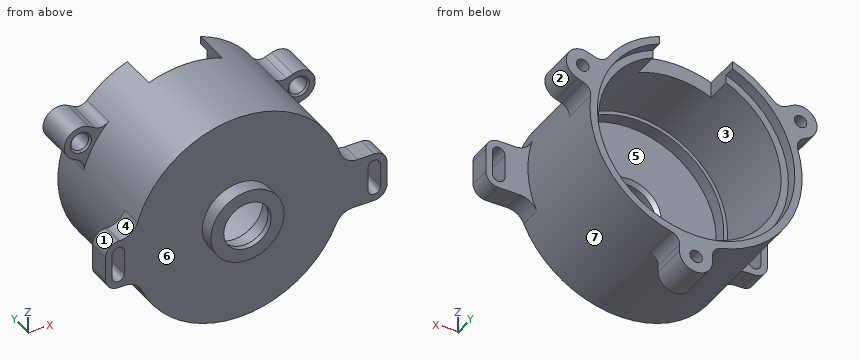
from build123d import *

# Parameters (mm, degrees)
ESQUISSE1_R                        = 2.4
BOSS_EXTRU_1_DEPTH                 = 10
ESQUISSE1_3_R                      = 2.4
BOSS_EXTRU_2_DEPTH                 = 4
CHANFREIN2_SIZE                    = 0.5
CONG_1_R                           = 3
R_P_TITION_START                   = 27.5
R_P_TITION_CIRCULAIRE1_OUTLINE_R   = 2.4
R_P_TITION_CIRCULAIRE1_DEPTH       = 4
R_P_TITION_START_2                 = 21.5
R_P_TITION_CIRCULAIRE1_2_OUTLINE_R = 2.4
R_P_TITION_CIRCULAIRE1_2_DEPTH     = 10
M3_CLEARANCE_HOLE1_D               = 3.4
ENL_V_MAT_EXTRU_2_DEPTH            = 10
BOSS_EXTRU_3_START                 = -6
BOSS_EXTRU_3_DEPTH                 = 6
CONG_3_R                           = 5


with BuildPart() as part:
    # Sketch1 → Revolve1 (revolve)
    with BuildSketch(Plane.XY, mode=Mode.PRIVATE) as revolve1_sk:
        Polygon((29, -3.5), (29, 31.5), (27, 31.5), (27, 28.5), (25, 28.5), (25, 3.5), (24, 3.5), (24, 0), (9, 0), (8, -1), (8, -6), (6.5, -6), (6.5, -7.5), (10, -7.5), (10, -3.5), align=None)
    revolve(revolve1_sk.sketch.rotate(Axis((0, 34.575175177, 0), (0, -1, 0)), 90), axis=Axis((0, 34.575175177, 0), (0, -1, 0)))

    # Esquisse1 → Boss.-Extru.1 (add)
    with BuildSketch(Plane(origin=(0, 31.5, 0), x_dir=(1, 0, 0), z_dir=(0, 1, 0))):
        with BuildLine():
            Line((4.5, 28.648734702), (4.5, 33))
            ThreePointArc((4.5, 33), (0, 37.5), (-4.5, 33))
            Line((-4.5, 33), (-4.5, 28.648734702))
            ThreePointArc((-4.5, 28.648734702), (0, 29), (4.5, 28.648734702))
        make_face()
        with Locations(Location((0, 33, 0), (0, 0, 270))):
            Circle(ESQUISSE1_R, mode=Mode.SUBTRACT)
    extrude(amount=-BOSS_EXTRU_1_DEPTH)

    # Esquisse1<3> → Boss.-Extru.2 (add)
    with BuildSketch(Plane(origin=(0, 31.5, 0), x_dir=(1, 0, 0), z_dir=(0, 1, 0))):
        with Locations(Location((0, 33, 0), (0, 0, 270))):
            Circle(ESQUISSE1_3_R)
    extrude(amount=-BOSS_EXTRU_2_DEPTH)

    # Chanfrein2
    chanfrein2_edges = [part.edges().sort_by_distance(p)[0] for p in [
        (0, 21.5, -35.4),
    ]]
    chamfer(chanfrein2_edges, length=CHANFREIN2_SIZE)

    # Congé1
    cong_1_edges = [part.edges().sort_by_distance(p)[0] for p in [
        (4.5, 26.5, -28.648734702),
        (-4.5, 26.5, -28.648734702),
    ]]
    fillet(cong_1_edges, radius=CONG_1_R)



with BuildPart() as body_2:
    # Répétition circulaire1: read off the stored shape, not the designer's step
    # Répétition circulaire1 outline → Répétition circulaire1 (new body)
    with BuildSketch(Plane(origin=(0, 0, 0), x_dir=(1, 0, 0), z_dir=(0, 1, 0)).offset(R_P_TITION_START)):
        with Locations((31.009856486, -11.28666473)):
            Circle(R_P_TITION_CIRCULAIRE1_OUTLINE_R)
        with Locations((-28.578838325, -16.5)):
            Circle(R_P_TITION_CIRCULAIRE1_OUTLINE_R)
    extrude(amount=R_P_TITION_CIRCULAIRE1_DEPTH)


with BuildPart() as part_1:
    add(part.part)

    add(body_2.part)  # R_p_tition circulaire1 2 merges body 2
    # R_p_tition circulaire1 2 outline → R_p_tition circulaire1 2 (add)
    # profile 1 of 2: a face of its own
    with BuildSketch(Plane(origin=(0, 0, 0), x_dir=(1, 0, 0), z_dir=(0, 1, 0)).offset(R_P_TITION_START_2)):
        with BuildLine():
            Line((-29.190907557, -11.657225913), (-30.828838325, -12.602885683))
            ThreePointArc((-30.828838325, -12.602885683), (-32.475952642, -18.75), (-26.328838325, -20.397114317))
            Line((-26.328838325, -20.397114317), (-24.690907557, -19.451454547))
            ThreePointArc((-24.690907557, -19.451454547), (-22.761849141, -19.080371134), (-21.016759974, -19.98238725))
            ThreePointArc((-21.016759974, -19.98238725), (-25.11473671, -14.5), (-27.813634974, -8.209854417))
            ThreePointArc((-27.813634974, -8.209854417), (-27.905010686, -10.172154026), (-29.190907557, -11.657225913))
        make_face()
        with Locations((-28.578838325, -16.5)):
            Circle(R_P_TITION_CIRCULAIRE1_2_OUTLINE_R, mode=Mode.SUBTRACT)
    # profile 2 of 2: a face of its own
    with BuildSketch(Plane(origin=(0, 0, 0), x_dir=(1, 0, 0), z_dir=(0, 1, 0)).offset(R_P_TITION_START_2)):
        with BuildLine():
            ThreePointArc((30.771688116, -6.411178556), (29.247446881, -5.171961896), (28.81670962, -3.255341254))
            ThreePointArc((28.81670962, -3.255341254), (27.251086003, -9.918584157), (24.167373297, -16.029287818))
            ThreePointArc((24.167373297, -16.029287818), (25.729317183, -14.8379438), (27.693506826, -14.868412143))
            Line((27.693506826, -14.868412143), (29.470765841, -15.515281523))
            ThreePointArc((29.470765841, -15.515281523), (35.238473279, -12.825755374), (32.548947131, -7.058047936))
            Line((32.548947131, -7.058047936), (30.771688116, -6.411178556))
        make_face()
        with Locations((31.009856486, -11.28666473)):
            Circle(R_P_TITION_CIRCULAIRE1_2_OUTLINE_R, mode=Mode.SUBTRACT)
    extrude(amount=R_P_TITION_CIRCULAIRE1_2_DEPTH)

    # R_p_tition circulaire1 3: loft between two sections, ruled curve by curve
    r_p_tition_circulaire1_3_from = [
        Edge.make_three_point_arc((-28.578838325, 22, 18.9), (-30.978838325, 22, 16.5), (-28.578838325, 22, 14.1)),
        Edge.make_three_point_arc((-28.578838325, 22, 14.1), (-26.178838325, 22, 16.5), (-28.578838325, 22, 18.9)),
    ]
    r_p_tition_circulaire1_3_to = [
        Edge.make_three_point_arc((-28.578838325, 21.5, 19.4), (-31.478838325, 21.5, 16.5), (-28.578838325, 21.5, 13.6)),
        Edge.make_three_point_arc((-28.578838325, 21.5, 13.6), (-25.678838325, 21.5, 16.5), (-28.578838325, 21.5, 19.4)),
    ]
    r_p_tition_circulaire1_3 = Solid(Shell([*[Face.make_surface_from_curves(r_p_tition_circulaire1_3_from[k], r_p_tition_circulaire1_3_to[k]) for k in range(2)], Face(Wire(r_p_tition_circulaire1_3_from)), Face(Wire(r_p_tition_circulaire1_3_to))]))
    add(r_p_tition_circulaire1_3, mode=Mode.SUBTRACT)

    # R_p_tition circulaire1 4: loft between two sections, ruled curve by curve
    r_p_tition_circulaire1_4_from = [
        Edge.make_three_point_arc((31.009856486, 22, 13.68666473), (28.609856486, 22, 11.28666473), (31.009856486, 22, 8.88666473)),
        Edge.make_three_point_arc((31.009856486, 22, 8.88666473), (33.409856486, 22, 11.28666473), (31.009856486, 22, 13.68666473)),
    ]
    r_p_tition_circulaire1_4_to = [
        Edge.make_three_point_arc((31.009856486, 21.5, 14.18666473), (28.109856486, 21.5, 11.28666473), (31.009856486, 21.5, 8.38666473)),
        Edge.make_three_point_arc((31.009856486, 21.5, 8.38666473), (33.909856486, 21.5, 11.28666473), (31.009856486, 21.5, 14.18666473)),
    ]
    r_p_tition_circulaire1_4 = Solid(Shell([*[Face.make_surface_from_curves(r_p_tition_circulaire1_4_from[k], r_p_tition_circulaire1_4_to[k]) for k in range(2)], Face(Wire(r_p_tition_circulaire1_4_from)), Face(Wire(r_p_tition_circulaire1_4_to))]))
    add(r_p_tition_circulaire1_4, mode=Mode.SUBTRACT)

    # M3 Clearance Hole1 (through all)
    with Locations(Plane(origin=(0, 31.5, 0), x_dir=(1, 0, 0), z_dir=(0, 1, 0))):
        with Locations((0, 33), (-28.578838325, -16.5), (31.009856486, -11.28666473)):
            Hole(M3_CLEARANCE_HOLE1_D / 2)

    # Esquisse5 → Enlèv. mat.-Extru.2 (cut)
    with BuildSketch(Plane(origin=(0, 31.5, 0), x_dir=(1, 0, 0), z_dir=(0, 1, 0))):
        with BuildLine():
            Line((-10, -22.912878475), (-10, -27.221315178))
            ThreePointArc((-10, -27.221315178), (0, -29), (10, -27.221315178))
            Line((10, -27.221315178), (10, -22.912878475))
            ThreePointArc((10, -22.912878475), (0, -25), (-10, -22.912878475))
        make_face()
    extrude(amount=-ENL_V_MAT_EXTRU_2_DEPTH, mode=Mode.SUBTRACT)

    # Esquisse6 → Boss.-Extru.3 (add)
    # profile 1 of 4: a face of its own
    with BuildSketch(Plane.XZ.offset(3.5).offset(BOSS_EXTRU_3_START)):
        with BuildLine():
            Line((37, 5), (28.565713714, 5))
            ThreePointArc((28.565713714, 5), (28.891224426, 2.50941251), (29, 0))
            ThreePointArc((29, 0), (28.679817788, -4.297447108), (27.726341266, -8.5))
            Line((27.726341266, -8.5), (37, -8.5))
            ThreePointArc((37, -8.5), (34.525126266, -7.474873734), (33.5, -5))
            Line((33.5, -5), (33.5, 1.5))
            ThreePointArc((33.5, 1.5), (34.525126266, 3.974873734), (37, 5))
        make_face()
    # profile 2 of 4: a face of its own
    with BuildSketch(Plane.XZ.offset(3.5).offset(BOSS_EXTRU_3_START)):
        with BuildLine():
            ThreePointArc((33.5, -5), (37, -8.5), (40.5, -5))
            Line((40.5, -5), (40.5, 1.5))
            ThreePointArc((40.5, 1.5), (37, 5), (33.5, 1.5))
            Line((33.5, 1.5), (33.5, -5))
        make_face()
        with BuildLine():
            ThreePointArc((38.7, 1.5), (37, 3.2), (35.3, 1.5))
            Line((35.3, 1.5), (35.3, -5))
            ThreePointArc((35.3, -5), (37, -6.7), (38.7, -5))
            Line((38.7, -5), (38.7, 1.5))
        make_face(mode=Mode.SUBTRACT)
    # profile 3 of 4: a face of its own
    with BuildSketch(Plane.XZ.offset(3.5).offset(BOSS_EXTRU_3_START)):
        with BuildLine():
            ThreePointArc((-33, 5), (-30.525126266, 3.974873734), (-29.5, 1.5))
            Line((-29.5, 1.5), (-29.5, -5))
            ThreePointArc((-29.5, -5), (-30.525126266, -7.474873734), (-33, -8.5))
            Line((-33, -8.5), (-27.726341266, -8.5))
            ThreePointArc((-27.726341266, -8.5), (-28.944107578, -1.799621218), (-28.565713714, 5))
            Line((-28.565713714, 5), (-33, 5))
        make_face()
    # profile 4 of 4: a face of its own
    with BuildSketch(Plane.XZ.offset(3.5).offset(BOSS_EXTRU_3_START)):
        with BuildLine():
            ThreePointArc((-36.5, -5), (-33, -8.5), (-29.5, -5))
            Line((-29.5, -5), (-29.5, 1.5))
            ThreePointArc((-29.5, 1.5), (-33, 5), (-36.5, 1.5))
            Line((-36.5, 1.5), (-36.5, -5))
        make_face()
        with BuildLine():
            ThreePointArc((-31.3, 1.5), (-33, 3.2), (-34.7, 1.5))
            Line((-34.7, 1.5), (-34.7, -5))
            ThreePointArc((-34.7, -5), (-33, -6.7), (-31.3, -5))
            Line((-31.3, -5), (-31.3, 1.5))
        make_face(mode=Mode.SUBTRACT)
    extrude(amount=BOSS_EXTRU_3_DEPTH)

    # Congé3
    cong_3_edges = [part_1.edges().sort_by_distance(p)[0] for p in [
        (27.726341266, -0.5, -8.5),
        (28.565713714, -0.5, 5),
        (-28.565713714, -0.5, 5),
        (-27.726341266, -0.5, -8.5),
    ]]
    fillet(cong_3_edges, radius=CONG_3_R)


solid = part_1.part
The listing builds one solid part. Answer for the finished solid, in the listing's coordinates (mm). Face numbers are marked on the shaded views. A direction names the side the tool comes from. Give positions to 0.01 mm unless a question says otherwise; leave off trailing zeros. Write each loop counter-clockwise with the first axis right and the second up, starting at its lowest first coordinate (ties: lowest second). Pieces come first, ordered by that corner, then holes. Notation, with made-up numbers: (-35.75, 55) - (18.25, 55) arc R32 ccw to (18.25, 88) - close; hole circle Ø10 at (-28, 10.5). An arc over 180 degrees is marked (long way). One line per question, with ' | ' between items. Start each with the question number.
1. Straight lines are drawn through the part: line 1 (X direction, y = 28.55, z = -33); line 2 (X direction, y = 30.55, z = 0); line 3 (Z direction, x = 0, y = 29.6). For each, find the intervals that lie inside material, in ascending order.
2. Section A-A, the plane x = 0 is taken. Count the separate pieces of the cut face and the enclosed holes in it, then the cut area to 3 significant figures.
3. Determine the mould class of the marked faces 1, 2 and 3 for opening direction Z: +Z half, -Z half, draft (parallel to the pull), parting line (faces both ways), or undercut.
4. For the marked faces 4, 5, 6 and 7, determine the directions among +Z, -Z, +X, -X, +Y, -Y from which every point of the face is accessible in a straight line to the end or side of a thin tool.
5. Given P1, Ø5.5, axis at x = 1, z = -33, coming from the -Y side; P2, Ø5.5, axis at x = -28.58, z = 16.5, coming from the -Y side; P3, Ø8, axis at x = 14.5, z = -20.5, coming from the -Y side, each flat-ended and moving along its own axis, determine where each tip first touches the part or whether it passes through.
6. Section B-B, the plane y = 8 is taken. Determine the outline of the cut face in (x, z).
7. Section D-D, the plane z = -16 is taken. Determine the outline of the cut face in (x, y).
Result:
1) line 1: x = -4.5 to -1.7, 1.7 to 4.5 | line 2: x = -29 to -27, 27 to 29 | line 3: z = -37.5 to -34.7, -31.3 to -27
2) separate pieces: 3 | enclosed holes: 0 | area: 422 mm2
3) face 1: +Z half | face 2: parting line | face 3: undercut
4) face 4: +Z, -X, +Y, -Y | face 5: +Y | face 6: -Y | face 7: none
5) P1: stops at y = 21.5 | P2: stops at y = 21.65 | P3: stops at y = -3.5
6) outline: circle Ø58 at (0, 0); hole circle Ø50 at (0, 0)
7) outline: (-24.19, -3.5) - (24.19, -3.5) - (24.19, 31.5) - (21.75, 31.5) - (21.75, 28.5) - (19.21, 28.5) - (19.21, 3.5) - (17.89, 3.5) - (17.89, 0) - (-17.89, 0) - (-17.89, 3.5) - (-19.21, 3.5) - (-19.21, 28.5) - (-21.75, 28.5) - (-21.75, 31.5) - (-24.19, 31.5) - close
